```python
from build123d import *

# Parameters (mm, degrees)
SKETCH1_W                                    = 100
SKETCH1_H                                    = 100
BOSS_EXTRUDE1_DEPTH                          = 3
SKETCH4_R                                    = 5
BOSS_EXTRUDE2_DEPTH                          = 5
SKETCH6_R                                    = 5
BOSS_EXTRUDE3_DEPTH                          = 5
SKETCH5_R                                    = 1.325
SKETCH5_R_2                                  = 1.15
CUT_EXTRUDE1_DEPTH                           = 9
SKETCH7_W                                    = 80
SKETCH7_H                                    = 40
CUT_EXTRUDE2_DEPTH                           = 4
FILLET2_R                                    = 5
CSK_FOR_M4_COUNTERSUNK_FLAT_HEAD_SCR_2_COUNT = 2
CSK_FOR_M4_COUNTERSUNK_FLAT_HEAD_SCR_2_PITCH = 16
CSK_FOR_M4_COUNTERSUNK_FLAT_HEAD_SCR_3_COUNT = 2
CSK_FOR_M4_COUNTERSUNK_FLAT_HEAD_SCR_3_PITCH = 22.627416998
CSK_FOR_M4_COUNTERSUNK_FLAT_HEAD_SCR_4_COUNT = 2
CSK_FOR_M4_COUNTERSUNK_FLAT_HEAD_SCR_4_PITCH = 35.77708764
CSK_FOR_M4_COUNTERSUNK_FLAT_HEAD_SCR_5_COUNT = 2
CSK_FOR_M4_COUNTERSUNK_FLAT_HEAD_SCR_5_PITCH = 32


with BuildPart() as part:
    # Sketch1 → Boss-Extrude1 (new body)
    with BuildSketch(Plane(origin=(0, 0, 0), x_dir=(1, 0, 0), z_dir=(0, 1, 0))):
        Rectangle(SKETCH1_W, SKETCH1_H)
    extrude(amount=BOSS_EXTRUDE1_DEPTH)

    # Sketch4 → Boss-Extrude2 (add)
    with BuildSketch(Plane(origin=(0, 3, 0), x_dir=(1, 0, 0), z_dir=(0, 1, 0))):
        with Locations((-45, 45)):
            Circle(SKETCH4_R)
        with Locations((-45, -5)):
            Circle(SKETCH4_R)
        with Locations((45, -5)):
            Circle(SKETCH4_R)
        with Locations((45, 45)):
            Circle(SKETCH4_R)
    extrude(amount=BOSS_EXTRUDE2_DEPTH)

    # Sketch6 → Boss-Extrude3 (add)
    with BuildSketch(Plane(origin=(0, 3, 0), x_dir=(1, 0, 0), z_dir=(0, 1, 0))):
        with Locations((39.5, -44.75)):
            Circle(SKETCH6_R)
        with Locations((39.5, -14.75)):
            Circle(SKETCH6_R)
        with Locations((9.5, -44.75)):
            Circle(SKETCH6_R)
        with Locations((-0.5, -14.75)):
            Circle(SKETCH6_R)
        with Locations((-35, -28)):
            Circle(SKETCH6_R)
        with Locations((-15, -43)):
            Circle(SKETCH6_R)
    extrude(amount=BOSS_EXTRUDE3_DEPTH)

    # Sketch5 → Cut-Extrude1 (cut, through all)
    with BuildSketch(Plane(origin=(0, 8, 0), x_dir=(1, 0, 0), z_dir=(0, 1, 0))):
        with Locations((-45, 45)):
            Circle(SKETCH5_R)
        with Locations((45, 45)):
            Circle(SKETCH5_R)
        with Locations((45, -5)):
            Circle(SKETCH5_R)
        with Locations((-45, -5)):
            Circle(SKETCH5_R)
        with Locations((39.5, -14.75)):
            Circle(SKETCH5_R_2)
        with Locations((39.5, -44.75)):
            Circle(SKETCH5_R_2)
        with Locations((9.5, -44.75)):
            Circle(SKETCH5_R_2)
        with Locations((-0.5, -14.75)):
            Circle(SKETCH5_R_2)
        with Locations((-35, -28)):
            Circle(SKETCH5_R)
        with Locations((-15, -43)):
            Circle(SKETCH5_R)
    extrude(amount=-CUT_EXTRUDE1_DEPTH, mode=Mode.SUBTRACT)

    # Sketch7 → Cut-Extrude2 (cut, through all)
    with BuildSketch(Plane(origin=(0, 3, 0), x_dir=(1, 0, 0), z_dir=(0, 1, 0))):
        with Locations((0, 20)):
            Rectangle(SKETCH7_W, SKETCH7_H)
    extrude(amount=-CUT_EXTRUDE2_DEPTH, mode=Mode.SUBTRACT)

    # Fillet2
    fillet2_edges = [part.edges().sort_by_distance(p)[0] for p in [
        (50, 1.5, -50),
        (-50, 1.5, -50),
        (-50, 1.5, 50),
        (50, 1.5, 50),
        (40, 1.5, 0),
        (40, 1.5, -40),
        (-40, 1.5, -40),
        (-40, 1.5, 0),
    ]]
    fillet(fillet2_edges, radius=FILLET2_R)

    # Sketch11 → CSK for M4 Countersunk Flat Head Screw1 (revolve, cut)
    with BuildSketch(Plane(origin=(-16, 3, 12.372677549), x_dir=(0, 0, 1), z_dir=(1, 0, 0))):
        Polygon((0, 0), (0, 3), (2.25, 3), (2.25, 2.45), (4.7, 0), align=None)
    csk_for_m4_countersunk_flat_head_screw1 = revolve(axis=Axis((-16, 9.35, 12.372677549), (0, -1, 0)), mode=Mode.SUBTRACT)

    # CSK for M4 Countersunk Flat Head Scr 2: CSK for M4 Countersunk Flat Head Screw1 ×2
    with Locations(*[(0, 0, i * CSK_FOR_M4_COUNTERSUNK_FLAT_HEAD_SCR_2_PITCH) for i in range(1, CSK_FOR_M4_COUNTERSUNK_FLAT_HEAD_SCR_2_COUNT)]):
        add(csk_for_m4_countersunk_flat_head_screw1, mode=Mode.SUBTRACT)

    # CSK for M4 Countersunk Flat Head Scr 3: CSK for M4 Countersunk Flat Head Screw1 ×2
    with Locations(*[Vector(0.707106781, 0, 0.707106781) * (i * CSK_FOR_M4_COUNTERSUNK_FLAT_HEAD_SCR_3_PITCH) for i in range(1, CSK_FOR_M4_COUNTERSUNK_FLAT_HEAD_SCR_3_COUNT)]):
        add(csk_for_m4_countersunk_flat_head_screw1, mode=Mode.SUBTRACT)

    # CSK for M4 Countersunk Flat Head Scr 4: CSK for M4 Countersunk Flat Head Screw1 ×2
    with Locations(*[Vector(0.894427191, 0, 0.447213595) * (i * CSK_FOR_M4_COUNTERSUNK_FLAT_HEAD_SCR_4_PITCH) for i in range(1, CSK_FOR_M4_COUNTERSUNK_FLAT_HEAD_SCR_4_COUNT)]):
        add(csk_for_m4_countersunk_flat_head_screw1, mode=Mode.SUBTRACT)

    # CSK for M4 Countersunk Flat Head Scr 5: CSK for M4 Countersunk Flat Head Screw1 ×2
    with Locations(*[(i * CSK_FOR_M4_COUNTERSUNK_FLAT_HEAD_SCR_5_PITCH, 0, 0) for i in range(1, CSK_FOR_M4_COUNTERSUNK_FLAT_HEAD_SCR_5_COUNT)]):
        add(csk_for_m4_countersunk_flat_head_screw1, mode=Mode.SUBTRACT)


solid = part.part
```
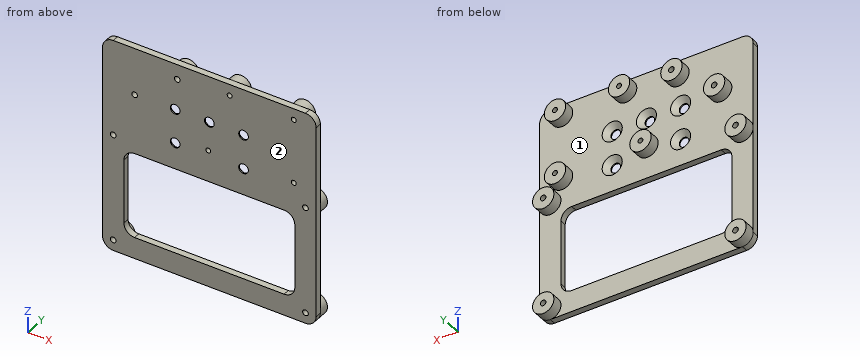
Work out the finished part from the listing and answer in its coordinate system (mm). Face numbers are marked on the shaded views. A direction names the side the tool comes from. Round coordinates to 2 decimals unless told otherwise and drop trailing zeros. Loops run counter-clockwise (first coordinate to the right, second up) from the corner with the lowest first, then second, coordinate; pieces in that order, holes last. Notation, with made-up numbers: M 44.25,-16 L 87.25,-16 A12 ccw 87.25,-11 Z; hole C 8,-30 d3. An arc over 180 degrees is marked long. One line per question, with ' | ' between items.
Q1. Find section C-C, the plane x = 27. Give the vertices of the cut face in (y, z), then the cut area to 3 significant figures.
Conclusion:
outline: M 0,-50 L 3,-50 L 3,-40 L 0,-40 Z; M 0,0 L 3,0 L 3,50 L 0,50 Z | area: 180 mm2
Q2. Each of these flat-tipped pins is pushed along its axis until it touches: pin 1 Ø1.4 at (x, z) = (-0.5, 14.75) entering from +Y; pin 2 Ø2 at (x, z) = (-39, 12) entering from +Y; pin 3 Ø1.5 at (y, z) = (5, 18.5) entering from +X; pin 4 Ø6 at (x, z) = (-16, 12.37) entering from +Y. Where does it stop, or does it pass through?
Conclusion:
pin 1: passes through | pin 2: stops at y = 3 | pin 3: stops at x = 43.5 | pin 4: stops at y = 1.3
Q3. A tool of negligible diameter and unlimited length cuts with its end or side. For the marked faces 1 and 2, from which of +Z, -Z, +X, -X, +Y, -Y can it reach the whole face along a straight path? Write none if from no direction.
Conclusion:
face 1: +Y | face 2: +Z, -Z, +X, -X, -Y
Q4. Consider line 1 along X through (y, z) = (6, 5) (3 decimals); line 2 along Z through (x, y) = (-45, 1.75) (3 decimals); line 3 along X through (y, z) = (2, 45). Determine where each line is inside the solid, lowest interval first. Write a range as from..to.
Conclusion:
line 1: x = -50..-46.325, -43.675..-40, 40..43.675, 46.325..50 | line 2: z = -50..-46.325, -43.675..3.675, 6.325..50 | line 3: x = -50..8.38, 10.62..38.38, 40.62..50
Q5. Find section B-B, the plane z = -15. Give the vertices of the cut face in (x, y), then the cut area to 3 significant figures.
Conclusion:
outline: M -50,0 L -40,0 L -40,3 L -50,3 Z; M 40,0 L 50,0 L 50,3 L 40,3 Z | area: 60.0 mm2
Q6. Find section A-A, the plane y = 4.75. State how many separate pieces and enclosed holes the cut face has, then the cut area to 3 significant figures.
Conclusion:
separate pieces: 10 | enclosed holes: 10 | area: 736 mm2
Q7. Find section D-D, the plane x = 9.5. Give the vertices of the cut face in (y, z).
Conclusion:
outline: M 0,-50 L 3,-50 L 3,-40 L 0,-40 Z; M 0,0 L 3,0 L 3,39.75 L 8,39.75 L 8,43.6 L 0,43.6 Z; M 0,45.9 L 8,45.9 L 8,49.75 L 3,49.75 L 3,50 L 0,50 Z
